from build123d import *

# Parameters (mm, degrees)
F0_R            = 2.15265
F0_R_2          = 4.7625
F0_W            = 9.525
F0_H            = 3.175
F1_DEPTH        = 9.525
F2_R            = 2.15265
F3_REACH        = 44.1896136501
F6_R            = 3.96875
F7_DEPTH        = 6.35
F9_DEPTH        = 9.525
F9_COPIES_COUNT = 3
F9_COPIES_ANGLE = 180
F10_R           = 0.762
F12_R           = 3.96875
F13_DEPTH       = 6.35


# Not quite as in the source:
# - a feature of the source that left no trace in its solid (it failed there, or was rolled back) is left out
# - a pattern or mirror of a feature is missing from the dataset's text; its kind, count and spacing are read off the source's solid


with BuildPart() as f1:
    # F0 (on Top) → F1 (new body)
    with BuildSketch(Plane.XY):
        with BuildLine():
            Line((3.96875, 15.875), (-3.96875, 15.875))
            Line((-3.96875, 15.875), (-3.96875, 21.8677764859))
            ThreePointArc((-3.96875, 21.8677764859), (0, -22.225), (3.96875, 21.8677764859))
            Line((3.96875, 21.8677764859), (3.96875, 15.875))
        make_face()
        with Locations((-11.7865861589, -11.7865861589)):
            Circle(F0_R, mode=Mode.SUBTRACT)
        with Locations((11.7865861589, -11.7865861589)):
            Circle(F0_R, mode=Mode.SUBTRACT)
        with Locations((-11.7865861589, 11.7865861589)):
            Circle(F0_R, mode=Mode.SUBTRACT)
        Circle(F0_R_2, mode=Mode.SUBTRACT)
        with Locations((0, 9.525)):
            Rectangle(F0_W, F0_H, mode=Mode.SUBTRACT)
        with Locations((11.7865861589, 11.7865861589)):
            Circle(F0_R, mode=Mode.SUBTRACT)
    extrude(amount=F1_DEPTH)

    f3_end = f1.faces().sort_by_distance((-4.7625, 0, 4.7625))[0]
    # F2 (on face) → F3 (cut, up to a face of the model that its end follows)
    with BuildSketch(Plane(origin=(0, 15.875, 0), x_dir=(-1, 0, 0), z_dir=(0, 1, 0))):
        with Locations((0, 4.7625)):
            Circle(F2_R)
    f3_long = extrude(amount=-F3_REACH, mode=Mode.PRIVATE)
    add(split(f3_long, bisect_by=f3_end, keep=Keep.ALL, mode=Mode.PRIVATE).solids().sort_by_distance((0, 15.875, 4.7625))[0], mode=Mode.SUBTRACT)

    # F6 (on face) → F7 (cut, through all)
    with BuildSketch(Plane(origin=(0, 0, 0), x_dir=(1, 0, 0), z_dir=(0, 0, -1))):
        with Locations((11.7865861589, -11.7865861589)):
            Circle(F6_R)
        with Locations((-11.7865861589, 11.7865861589)):
            Circle(F6_R)
    extrude(amount=-F7_DEPTH, mode=Mode.SUBTRACT)

    # F8 (on face) → F9 (cut, through all)
    with BuildSketch(Plane(origin=(0, 0, 0), x_dir=(1, 0, 0), z_dir=(0, 0, -1))):
        with BuildLine():
            ThreePointArc((-17.3148424047, -11.229543123), (-14.7565267097, -7.0906978311), (-9.9206262673, -6.5530302219))
            Line((-9.9206262673, -6.5530302219), (-7.0379344931, -3.6703384477))
            ThreePointArc((-7.0379344931, -3.6703384477), (-7.9375, 0), (-7.0379344931, 3.6703384477))
            Line((-7.0379344931, 3.6703384477), (-9.9206262673, 6.5530302219))
            ThreePointArc((-9.9206262673, 6.5530302219), (-14.7565267097, 7.0906978311), (-17.3148424047, 11.229543123))
            ThreePointArc((-17.3148424047, 11.229543123), (-20.6375, 0), (-17.3148424047, -11.229543123))
        make_face()
    f9 = extrude(amount=-F9_DEPTH, mode=Mode.SUBTRACT)

    # F9_copies: F9 ×3 about axis
    f9_copies_axis = Axis((0, 0, 0), (0, 0, 1))
    for i in range(1, F9_COPIES_COUNT):
        add(f9.rotate(f9_copies_axis, i * F9_COPIES_ANGLE / (F9_COPIES_COUNT - 1)), mode=Mode.SUBTRACT)

    # F10
    f10_edges = [f1.edges().sort_by_distance(p)[0] for p in [
        (-17.314842, -11.229543, 4.7625),
        (-9.920626, -6.55303, 4.7625),
        (-7.037934, -3.670338, 4.7625),
        (-7.037934, 3.670338, 4.7625),
        (-9.920626, 6.55303, 4.7625),
        (-17.314842, 11.229543, 4.7625),
        (3.96875, 21.867776, 4.7625),
        (-3.96875, 21.867776, 4.7625),
        (11.229543, -17.314842, 4.7625),
        (-11.229543, -17.314842, 4.7625),
        (6.55303, -9.920626, 4.7625),
        (-6.55303, -9.920626, 4.7625),
        (3.670338, -7.037934, 4.7625),
        (-3.670338, -7.037934, 4.7625),
        (17.314842, 11.229543, 4.7625),
        (17.314842, -11.229543, 4.7625),
        (9.920626, 6.55303, 4.7625),
        (7.037934, 3.670338, 4.7625),
        (7.037934, -3.670338, 4.7625),
        (9.920626, -6.55303, 4.7625),
    ]]
    fillet(f10_edges, radius=F10_R)

    # F12 (on face) → F13 (cut, through all)
    with BuildSketch(Plane.XY.offset(9.525)):
        with Locations((11.7865861589, -11.7865861589)):
            Circle(F12_R)
        with Locations((-11.7865861589, 11.7865861589)):
            Circle(F12_R)
    extrude(amount=-F13_DEPTH, mode=Mode.SUBTRACT)


solid = f1.part
CAD build for the part. Positions are in the model's coordinates, mm. A direction names the side the tool comes from. Give positions to 0.01 mm unless a question says otherwise; leave off trailing zeros. Write each loop counter-clockwise with the first axis right and the second up, starting at its lowest first coordinate (ties: lowest second). Pieces come first, ordered by that corner, then holes. Notation, with made-up numbers: (21, -23) -> (39, -23) arc R17 cw to (39, 8) -> close; hole circle Ø7 at (34, 32). An arc over 180 degrees is marked (long way). Return JSON: item names as keys, results as strings.
Item 1: Band-saw the part on B-B (y = 7). List the corners of the cut face in (x, z) (1 decimal), then the cut area to 3 significant figures.
Answer below:
{"outline": "(-21.1, 0) -> (-19.4, 0) -> (-19.4, 9.5) -> (-21.1, 9.5) -> close; (-14.6, 0) -> (14.6, 0) -> (14.6, 9.5) -> (-14.6, 9.5) -> close; (19.4, 0) -> (21.1, 0) -> (21.1, 9.5) -> (19.4, 9.5) -> close; hole circle Ø4.3 at (0, 4.8)", "area": "296 mm2"}
Item 2: Band-saw the part on D-D (y = -15). List the corners of the cut face in (x, z) (3 decimals), then the cut area to 3 significant figures.
Answer below:
{"outline": "(-16.4, 0) -> (-14.116, 0) -> (-14.116, 6.35) -> (-9.457, 6.35) -> (-9.457, 0) -> (-7.254, 0) -> (-7.254, 9.525) -> (-16.4, 9.525) -> close; (7.254, 0) -> (16.4, 0) -> (16.4, 9.525) -> (14.116, 9.525) -> (14.116, 3.175) -> (9.457, 3.175) -> (9.457, 9.525) -> (7.254, 9.525) -> close", "area": "115 mm2"}
Item 3: Drill centre lines: probe 1 along X at (y, z) = (11.5, 5.5); probe 2 along X at (y, z) = (15, 3); probe 3 along Y at (x, z) = (10.5, 1). Where is each one in solid material? Low to high.
Answer below:
{"probe 1": "x = -19.02 to -15.74, -7.83 to -2.02, 2.02 to 7.83, 15.74 to 19.02", "probe 2": "x = -16.4 to -1.24, 1.24 to 9.46, 14.12 to 16.4", "probe 3": "y = -19.59 to -13.51, -10.06 to -6.38, 6.38 to 8.03, 15.54 to 19.59"}
Item 4: Band-saw the part on C-C (y = 0). List the corners of the cut face in (x, z) (1 decimal), then the cut area to 3 significant figures.
Answer below:
{"outline": "(-22.2, 0) -> (-20.6, 0) -> (-20.6, 9.5) -> (-22.2, 9.5) -> close; (-7.9, 0) -> (-4.8, 0) -> (-4.8, 9.5) -> (-7.9, 9.5) -> close; (4.8, 0) -> (7.9, 0) -> (7.9, 9.5) -> (4.8, 9.5) -> close; (20.6, 0) -> (22.2, 0) -> (22.2, 9.5) -> (20.6, 9.5) -> close", "area": "90.7 mm2"}
Item 5: Drop flat-ended pins along their axis: pin 1 (5 mm diameter, centred on x = 0, z = 5, fed in from -Y) (3 decimals); pin 2 (2.5 mm diameter, centred on x = 0, z = 4.76, fed in from +Y); pin 3 (1.5 mm diameter, centred on y = 19.5, z = 5.5, fed in from +X); pin 4 (3.5 mm diameter, centred on x = -11.79, y = 11.79, fed in from +Z). Give the stop position or say it passes through.
Answer below:
{"pin 1": "stops at y = -22.225", "pin 2": "stops at y = -4.6", "pin 3": "stops at x = 11.93", "pin 4": "passes through"}
Item 6: Band-saw the part on A-A (x = 0). List the corners of the cut face in (y, z) (1 decimal).
Answer below:
{"outline": "(-22.2, 0) -> (-20.6, 0) -> (-20.6, 9.5) -> (-22.2, 9.5) -> close; (-7.9, 0) -> (-4.8, 0) -> (-4.8, 9.5) -> (-7.9, 9.5) -> close; (4.8, 0) -> (7.9, 0) -> (7.9, 2.6) -> (4.8, 2.6) -> close; (4.8, 6.9) -> (7.9, 6.9) -> (7.9, 9.5) -> (4.8, 9.5) -> close; (11.1, 0) -> (15.9, 0) -> (15.9, 2.6) -> (11.1, 2.6) -> close; (11.1, 6.9) -> (15.9, 6.9) -> (15.9, 9.5) -> (11.1, 9.5) -> close"}
Item 7: Tool access for faces 4 (the flat face through (-10, -10, 6.35)), 5 (the flat face through (-1.1, 7.938, 2.6)), 6 (the flat face through (13.5, -13.5, 3.175)): list every direction of +Z, -Z, +X, -X, +Y, -Y with a clear straight run to the whole face (end or side of a thin tool).
Answer below:
{"face 4": "-Z", "face 5": "+Z, -Z", "face 6": "+Z"}
Item 8: Two-plate mould, pull along Y, no slides. Class faces 1 (the flat face through (0, 5, 9.525)), 2 (the flat face through (-0.8, 15.875, 2.6)), 3 (the cylindrical face through (-6.8, -14.24, 4.7)): +Y half, -Y half, draft (parallel to the pull), parting line (faces both ways), or undercut.
Answer below:
{"face 1": "draft", "face 2": "+Y half", "face 3": "undercut"}
